from build123d import *

# Parameters (mm, degrees)
PAD_DEPTH    = 9
SKETCH001_W  = 10.5
SKETCH001_H  = 11.6
POCKET_DEPTH = 5


with BuildPart() as part:
    # Sketch → Pad (new body, symmetric)
    with BuildSketch(Plane.YZ):
        Polygon((-4, 22.5), (-4, 20), (-4.75, 10), (-5.25, 10), (-5.25, 20), (-7.25, 20), (-7.25, 22.5), align=None)
    extrude(amount=PAD_DEPTH, both=True)

    # Sketch001 (on Face6 of Pad) → Pocket (cut)
    with BuildSketch(Plane(origin=(0, -7.25, 0), x_dir=(0, 0, -1), z_dir=(0, -1, 0))):
        with Locations((-17.25, 0)):
            Rectangle(SKETCH001_W, SKETCH001_H)
    extrude(amount=-POCKET_DEPTH, mode=Mode.SUBTRACT)

    # Sphere → Sphere (revolve)
    with BuildSketch(Plane(origin=(7.4, -7.25, 21.25), x_dir=(0, 0, 1), z_dir=(-1, 0, 0))):
        with BuildLine():
            ThreePointArc((0, -1.25), (1.25, 0), (0, 1.25))
            Line((0, 1.25), (0, -1.25))
        make_face()
    revolve(axis=Axis((7.4, -7.25, 21.25), (0, 1, 0)))

    # Sphere001 → Sphere001 (revolve)
    with BuildSketch(Plane(origin=(-7.4, -7.25, 21.25), x_dir=(0, 0, 1), z_dir=(-1, 0, 0))):
        with BuildLine():
            ThreePointArc((0, -1.25), (1.25, 0), (0, 1.25))
            Line((0, 1.25), (0, -1.25))
        make_face()
    revolve(axis=Axis((-7.4, -7.25, 21.25), (0, 1, 0)))


solid = part.part
Part model, mm, in its own coordinate system. A direction names the side the tool comes from. Coordinates: 2 decimals unless noted, no trailing zeros. Write each loop counter-clockwise with the first axis right and the second up, starting at its lowest first coordinate (ties: lowest second). Pieces come first, ordered by that corner, then holes. Notation, with made-up numbers: (51.25, 9.5) - (72.25, 9.5) arc R13 cw to (72.25, 19.5) - close; hole circle Ø9 at (11.25, 63.25). An arc over 180 degrees is marked (long way). Put each result on its own line as item: value.
1. Probe line 1 along X through (y, z) = (-4.45, 19.75); line 2 along X through (y, z) = (-7.6, 22); line 3 along Z through (x, y) = (-8, -5.9). List the from-to ranges inside material, lowest first. Write a range as [from, to].
Final values:
line 1: x = [-9, -5.8], [5.8, 9]
line 2: x = [-8.34, -6.46], [6.46, 8.34]
line 3: z = [20, 22.5]
2. Flat gauge pins, fed straight in: pin 1 Ø0.5 at (x, z) = (-8, 21.5) entering from -Y; pin 2 Ø2 at (x, y) = (-7, -6.5) entering from -Z; pin 3 Ø0.5 at (x, z) = (-6.5, 22) entering from -Y. Where does each tip first touch, or does it go through?
Final values:
pin 1: stops at y = -8.43
pin 2: stops at z = 20
pin 3: stops at y = -8.09
3. Two-plate mould, pull along X, no slides. Class faces 1 (the flat face through (-6, -7.25, 21)), 2 (the flat face through (-7, -4, 21)), 3 (the flat face through (-9, -5, 18)), 4 (the flat face through (6, -7.25, 21)): +X half, -X half, draft (parallel to the pull), parting line (faces both ways), or undercut.
Final values:
face 1: undercut
face 2: draft
face 3: -X half
face 4: undercut
4. Band-saw the part on B-B (y = -6.65). Write the cut outline in (x, z).
Final values:
outline: (-9, 20) - (-5.8, 20) - (-5.8, 22.5) - (-9, 22.5) - close; (5.8, 20) - (9, 20) - (9, 22.5) - (5.8, 22.5) - close
5. Band-saw the part on A-A (z = 20.5). Write the cut outline in (x, y).
Final values:
outline: (-9, -7.25) - (-8.4, -7.25) arc R1 ccw to (-6.4, -7.25) - (-5.8, -7.25) - (-5.8, -4) - (-9, -4) - close; (5.8, -7.25) - (6.4, -7.25) arc R1 ccw to (8.4, -7.25) - (9, -7.25) - (9, -4) - (5.8, -4) - close
6. Band-saw the part on D-D (x = -3). Write the cut outline in (y, z), then the cut area to 3 significant figures.
Final values:
outline: (-5.25, 10) - (-4.75, 10) - (-4.6, 12) - (-5.25, 12) - close
area: 1.15 mm²
7. Band-saw the part on C-C (z = 18). Write the cut outline in (x, y).
Final values:
outline: (-9, -5.25) - (-5.8, -5.25) - (-5.8, -4.15) - (-9, -4.15) - close; (5.8, -5.25) - (9, -5.25) - (9, -4.15) - (5.8, -4.15) - close
8. 3-axis set-ups, long thin cutter, end or side, ignore diameter. For faces 5 (the flat face through (0.13, -4.62, 11.74)), 6 (the flat face through (0.1, -5.25, 11.6)), 7 (the flat face through (-5.8, -5, 18)): which of +Z, -Z, +X, -X, +Y, -Y reach the whole face in a straight line?
Final values:
face 5: -Z, +X, -X, +Y
face 6: -Z, +X, -X, -Y
face 7: +Z, +Y, -Y
